from build123d import *

# Parameters (mm, degrees)
EXTRUDE_1_DEPTH     = 20
SKETCH_3_W          = 210
SKETCH_3_H          = 10
CUT_EXTRUDE_1_DEPTH = 15
SKETCH_4_W          = 160
SKETCH_4_H          = 5
CUT_EXTRUDE_2_DEPTH = 10
SKETCH_5_R          = 2.5
SKETCH_5_R_2        = 2
CUT_EXTRUDE_3_DEPTH = 10
CUT_EXTRUDE_4_DEPTH = 4.3
SKETCH_8_R          = 5.75
CUT_EXTRUDE_6_DEPTH = 15
CUT_EXTRUDE_7_DEPTH = 250.048188108
CUT_EXTRUDE_START   = -8
CUT_EXTRUDE_8_DEPTH = 8


with BuildPart() as part:
    # 草图1 → 凸台-拉伸1 (new body)
    with BuildSketch(Plane.XY):
        Polygon((-115, 220), (115, 220), (60, -50), (59.592592593, -52), (-59.592592593, -52), (-60, -50), align=None)
    extrude(amount=EXTRUDE_1_DEPTH)

    # 草图3 → 切除-拉伸1 (cut)
    with BuildSketch(Plane(origin=(0, 220, 0), x_dir=(1, 0, 0), z_dir=(0, 1, 0))):
        with Locations((0, -10)):
            Rectangle(SKETCH_3_W, SKETCH_3_H)
    extrude(amount=-CUT_EXTRUDE_1_DEPTH, mode=Mode.SUBTRACT)

    # 草图4 → 切除-拉伸2 (cut)
    with BuildSketch(Plane.XY.offset(20)):
        with Locations((0, 123.51)):
            Rectangle(SKETCH_4_W, SKETCH_4_H)
    extrude(amount=-CUT_EXTRUDE_2_DEPTH, mode=Mode.SUBTRACT)

    # 草图5 → 切除-拉伸3 (cut)
    with BuildSketch(Plane.XY.offset(20)):
        with Locations((-77.25, 205.6425573)):
            Circle(SKETCH_5_R)
        with Locations((-90, 186.5)):
            Circle(SKETCH_5_R)
        with Locations((-64.5, 186.5)):
            Circle(SKETCH_5_R)
        with Locations((-55, 104.1525573)):
            Circle(SKETCH_5_R_2)
        with Locations((-67.75, 85.01)):
            Circle(SKETCH_5_R_2)
        with Locations((-42.25, 85.01)):
            Circle(SKETCH_5_R_2)
        with Locations(Location((42.25, 85.01, 0), (0, 0, 180))):
            Circle(SKETCH_5_R_2)
        with Locations(Location((67.75, 85.01, 0), (0, 0, 180))):
            Circle(SKETCH_5_R_2)
        with Locations(Location((55, 104.1525573, 0), (0, 0, 180))):
            Circle(SKETCH_5_R_2)
        with Locations(Location((64.5, 186.5, 0), (0, 0, 180))):
            Circle(SKETCH_5_R)
        with Locations(Location((90, 186.5, 0), (0, 0, 180))):
            Circle(SKETCH_5_R)
        with Locations(Location((77.25, 205.6425573, 0), (0, 0, 345.106514196))):
            Circle(SKETCH_5_R)
    extrude(amount=-CUT_EXTRUDE_3_DEPTH, mode=Mode.SUBTRACT)

    # 草图6 → 切除-拉伸4 (cut, symmetric)
    with BuildSketch(Plane(origin=(0, 0, 10), x_dir=(-1, 0, 0), z_dir=(0, 0, -1))):
        with BuildLine():
            Line((0, -49.69), (17.486671343, -49.69))
            Line((17.486671343, -49.69), (12.108893566, -23.29))
            Line((12.108893566, -23.29), (0, -23.29))
            ThreePointArc((0, -23.29), (-13.2, -36.49), (0, -49.69))
        make_face()
    extrude(amount=CUT_EXTRUDE_4_DEPTH, both=True, mode=Mode.SUBTRACT)

    # 草图8 → 切除-拉伸6 (cut)
    with BuildSketch(Plane.XY.offset(20)):
        with Locations((0, -36.49)):
            Circle(SKETCH_8_R)
    extrude(amount=-CUT_EXTRUDE_6_DEPTH, mode=Mode.SUBTRACT)

    # 草图9 → 切除-拉伸7 (cut, through all)
    with BuildSketch(Plane.XY.offset(20)):
        with BuildLine():
            Line((13, 11.26), (47, 11.26))
            ThreePointArc((47, 11.26), (49.25, 13.51), (47, 15.76))
            Line((47, 15.76), (13, 15.76))
            ThreePointArc((13, 15.76), (10.75, 13.51), (13, 11.26))
        make_face()
    extrude(amount=-CUT_EXTRUDE_7_DEPTH, mode=Mode.SUBTRACT)

    # 草图10 → 切除-拉伸8 (cut)
    with BuildSketch(Plane(origin=(0, 0, 0), x_dir=(-1, 0, 0), z_dir=(0, 0, -1)).offset(CUT_EXTRUDE_START)):
        with BuildLine():
            Line((-50, 9.51), (-10, 9.51))
            ThreePointArc((-10, 9.51), (-6, 13.51), (-10, 17.51))
            Line((-10, 17.51), (-50, 17.51))
            ThreePointArc((-50, 17.51), (-54, 13.51), (-50, 9.51))
        make_face()
        with BuildLine():
            Line((-47, 15.76), (-13, 15.76))
            ThreePointArc((-13, 15.76), (-10.75, 13.51), (-13, 11.26))
            Line((-13, 11.26), (-47, 11.26))
            ThreePointArc((-47, 11.26), (-49.25, 13.51), (-47, 15.76))
        make_face(mode=Mode.SUBTRACT)
    extrude(amount=CUT_EXTRUDE_8_DEPTH, mode=Mode.SUBTRACT)


solid = part.part
Design review of the part built by this model. Coordinates are the model's own, in mm. A direction names the side the tool comes from. Give positions to 0.01 mm unless a question says otherwise; leave off trailing zeros. Order: outer loops, then holes, each group sorted by start corner. A loop starts at its lowest first (then second) coordinate and runs counter-clockwise, first axis right, second up. Notation, with made-up numbers: (12.5, 54) - (31.5, 54) arc R17 cw to (31.5, 76) - close; hole circle Ø9 at (82.25, 25.25). An arc over 180 degrees is marked (long way). Use CSV: the item, a comma, the result in double quotes. Start each with the question number.
Q1. Take a section at B-B (x = -33). State the section outline as (y, z) points.
Q2. For line 1 (Y direction, x = -42.25, z = 15.75); line 2 (Y direction, x = 55, z = 13.25); line 3 (Y direction, x = 38, z = 9), list the stretches that pass through material, from the lowest coordinate up.
Q3. Take a section at D-D (y = 179). State the section outline as (x, z) points, and give its area (3 significant figures).
Q4. Draft analysis for pull direction Y (two halves, no side actions). For faces 1 (the face through (1, -52, 10)), 2 (the face through (-9, -49.69, 10)), 3 (the face through (-1, 213, 15)), state which applies: pulls with the +Y half, pulls with the -Y half, needs draft (parallel to the pull), parting line crosses it, or undercut.
Q5. Machinability: for faces 4 (the face through (-1, 213, 5)), 5 (the face through (30, 15.76, 14)), 6 (the face through (-1, 121.01, 15)), 7 (the face through (-5.3, -39.2, 5.7)), 8 (the face through (6, 13.4, 4.1)), which of the approach directions +Z, -Z, +X, -X, +Y, -Y give a long, thin tool a straight path to every point of the face, cutting with its end or side? Answer none if there is none.
Q6. For P1, Ø8, axis at y = 213, z = 10.5, coming from the +X side; P2, Ø12, axis at y = -14, z = 8.5, coming from the +X side; P3, Ø4.5, axis at x = -13, z = 8, coming from the +Y side, all flat-tipped, find the tip position at first contact; note any pin that passes through.
Q7. Take a section at A-A (x = 30). State the section outline as (y, z) points, and give its area (3 significant figures).
Q8. Take a section at C-C (y = 141). State the section outline as (x, z) points, and give its area (3 significant figures).
Calculated:
1,outline,"(-52, 0) - (220, 0) - (220, 5) - (205, 5) - (205, 15) - (220, 15) - (220, 20) - (126.01, 20) - (126.01, 10) - (121.01, 10) - (121.01, 20) - (-52, 20) - close"
2,line 1,"y = -52 to 83.01, 87.01 to 121.01, 126.01 to 220"
2,line 2,"y = -52 to 102.15, 106.15 to 121.01, 126.01 to 205"
2,line 3,"y = -52 to 11.26, 15.76 to 205"
3,outline,"(-106.65, 0) - (106.65, 0) - (106.65, 20) - (-106.65, 20) - close"
3,area,"4,270 mm²"
4,face 1,"pulls with the -Y half"
4,face 2,"undercut"
4,face 3,"needs draft"
5,face 4,"+Y"
5,face 5,"+Z, -Z"
5,face 6,"+Z"
5,face 7,"none"
5,face 8,"-Z"
6,P1,"stops at x = 114.39"
6,P2,"stops at x = 68.56"
6,P3,"stops at y = 205"
7,outline,"(-52, 0) - (9.51, 0) - (9.51, 8) - (11.26, 8) - (11.26, 20) - (-52, 20) - close; (15.76, 8) - (17.51, 8) - (17.51, 0) - (220, 0) - (220, 5) - (205, 5) - (205, 15) - (220, 15) - (220, 20) - (126.01, 20) - (126.01, 10) - (121.01, 10) - (121.01, 20) - (15.76, 20) - close"
7,area,"5,120 mm²"
8,outline,"(-98.91, 0) - (98.91, 0) - (98.91, 20) - (-98.91, 20) - close"
8,area,"3,960 mm²"
